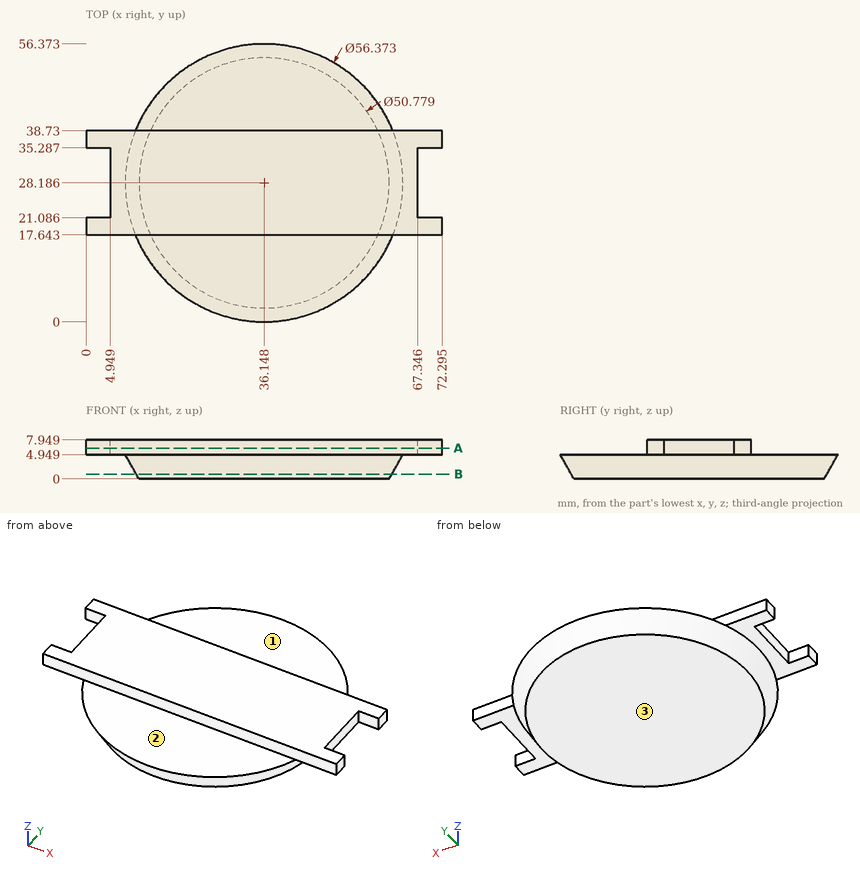
Part print with two shaded views. Sizes in mm from the minimum x, y, z corner. A direction names the side the tool comes from. Round coordinates to 2 decimals unless told otherwise and drop trailing zeros. Loops run counter-clockwise (first coordinate to the right, second up) from the corner with the lowest first, then second, coordinate; pieces in that order, holes last. Notation, with made-up numbers: (73, 33.5) - (111, 33.5) arc R31 cw to (111, 59.5) - close; hole circle Ø9 at (-10.75, 34). An arc over 180 degrees is marked (long way). Answer as a JSON object with one key per item and string values.
Item 1: Pin check, flat tips, straight feed: pin 1 (0.9 mm diameter, centred on x = 38.5, z = 6, fed in from -Y); pin 2 (3 mm diameter, centred on x = 65.5, y = 32, fed in from -Z) (1 decimal); pin 3 (1.5 mm diameter, centred on x = 20.5, z = 6, fed in from +Y). Stop position of each tip, or through.
Output:
{"pin 1": "y = 17.64", "pin 2": "z = 4.8", "pin 3": "y = 38.73"}
Item 2: Tool access for the marked faces 1, 2 and 3: list every direction of +Z, -Z, +X, -X, +Y, -Y with a clear straight run to the whole face (end or side of a thin tool).
Output:
{"face 1": "+Z, +X, -X, +Y", "face 2": "+Z, +X, -X, -Y", "face 3": "-Z, +X, -X, +Y, -Y"}
Item 3: Band-saw the part on A-A on z = 6.25. List the corners of the cut face in (x, y) (1 decimal), plus the area to 3 significant figures.
Output:
{"outline": "(0, 17.6) - (72.3, 17.6) - (72.3, 21.1) - (67.3, 21.1) - (67.3, 35.3) - (72.3, 35.3) - (72.3, 38.7) - (0, 38.7) - (0, 35.3) - (4.9, 35.3) - (4.9, 21.1) - (0, 21.1) - close", "area": "1,380 mm2"}
Item 4: Wall check: L1, parallel to Z at x = 42, y = 50; L2, parallel to X at y = 30, z = 5.75; L3, parallel to Y at x = 23, z = 7.5. Give the ranges that are in metal, low to high.
Output:
{"L1": "0 to 4.95", "L2": "4.95 to 67.35", "L3": "17.64 to 38.73"}
Item 5: Band-saw the part on B-B on z = 1. List the corners of the cut face in (x, y) (1 decimal).
Output:
{"outline": "circle Ø51.9 at (36.1, 28.2)"}
